Design review of the part built by this model. Coordinates are the model's own, in mm. Give positions to 0.01 mm unless a question says otherwise; leave off trailing zeros. Answer as CSV lines item,"result".
from build123d import *

# Parameters (mm, degrees)
SKETCH2_W           = 540
SKETCH2_H           = 10
BOSS_EXTRUDE1_DEPTH = 3
EXTRUDE_THIN1_DEPTH = 540


with BuildPart() as part:
    # Sketch2 → Boss-Extrude1 (new body)
    with BuildSketch(Plane.XY):
        with Locations((0, 5)):
            Rectangle(SKETCH2_W, SKETCH2_H)
    extrude(amount=BOSS_EXTRUDE1_DEPTH)

    # Sketch3 → Extrude-Thin1 (add, through all)
    with BuildSketch(Plane(origin=(270, 0, 0), x_dir=(0, 0, -1), z_dir=(1, 0, 0))):
        Polygon((0.193258825, -0.158590751), (8.206132428, 9.605903879), (16.412264855, -0.394096121), (24.618397283, 9.605903879), (32.824529711, -0.394096121), (41.030662139, 9.605903879), (49.236794566, -0.394096121), (57.442926994, 9.605903879), (65.649059422, -0.394096121), (73.85519185, 9.605903879), (82.061324277, -0.394096121), (90.267456705, 9.605903879), (98.473589133, -0.394096121), (106.679721561, 9.605903879), (114.885853988, -0.394096121), (123.091986416, 9.605903879), (131.298118844, -0.394096121), (139.504251272, 9.605903879), (147.710383699, -0.394096121), (155.916516127, 9.605903879), (164.122648555, -0.394096121), (172.328780983, 9.605903879), (180.53491341, -0.394096121), (188.741045838, 9.605903879), (196.947178266, -0.394096121), (205.153310694, 9.605903879), (213.166184296, -0.158590751), (213.552701947, 0.158590751), (205.153310694, 10.394096121), (196.947178266, 0.394096121), (188.741045838, 10.394096121), (180.53491341, 0.394096121), (172.328780983, 10.394096121), (164.122648555, 0.394096121), (155.916516127, 10.394096121), (147.710383699, 0.394096121), (139.504251272, 10.394096121), (131.298118844, 0.394096121), (123.091986416, 10.394096121), (114.885853988, 0.394096121), (106.679721561, 10.394096121), (98.473589133, 0.394096121), (90.267456705, 10.394096121), (82.061324277, 0.394096121), (73.85519185, 10.394096121), (65.649059422, 0.394096121), (57.442926994, 10.394096121), (49.236794566, 0.394096121), (41.030662139, 10.394096121), (32.824529711, 0.394096121), (24.618397283, 10.394096121), (16.412264855, 0.394096121), (8.206132428, 10.394096121), (-0.193258825, 0.158590751), align=None)
    extrude(amount=-EXTRUDE_THIN1_DEPTH)


solid = part.part
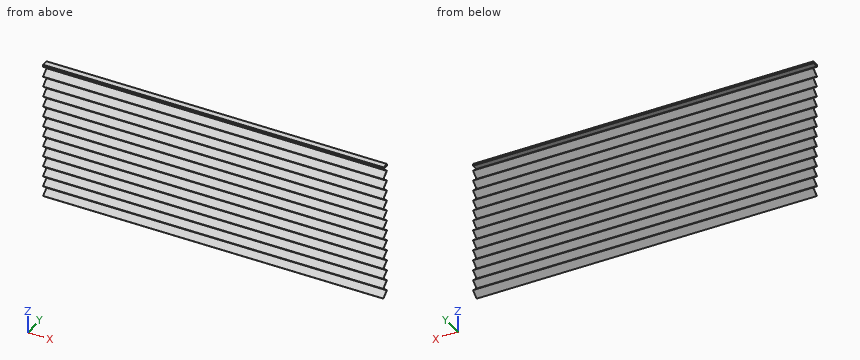
Q1. To check wall thickness, follow probe 1 along Y at (x, z) = (-31, -152); probe 2 along Y at (x, z) = (229, -196). State the ranges of each line that lie inside material, in increasing order. Write a range as from..to.
Filled sheet:
probe 1,"y = 4.83..5.62"
probe 2,"y = 0.76..1.55"
Q2. We need section A-A, the plane y = 7.5. State how many separate pieces and enclosed holes the cut face has, and give its area (3 significant figures).
Filled sheet:
separate pieces,"27"
enclosed holes,"0"
area,"10,700 mm^2"
Q3. Clearance check with flat-ended pins moving along their axes: pin 1 Ø4 at (x, z) = (120.5, -88) entering from +Y; pin 2 Ø4 at (x, z) = (-185, -119.5) entering from -Y; pin 3 Ø5 at (x, y) = (-13.5, 4) entering from -Z. State where each tip first meets the part, or that it passes through.
Filled sheet:
pin 1,"stops at y = 10.07"
pin 2,"stops at y = 2.79"
pin 3,"stops at z = -212.45"
